from build123d import *

# Parameters (mm, degrees)
SWEEP1_PROFILE_R     = 13.49375
CUT_SWEEP1_PROFILE_R = 9.525


with BuildPart() as part:
    # Sweep1: sweep along a curve in space
    with BuildLine() as sweep1_path:
        Line((-39.450636639, 0, 30.750046958), (-39.450636639, 0, 11.700046958))
        Line((-39.450636639, 0, 0), (-39.450636639, 0, 11.700046958))
        Line((-39.450636639, 0, -7.349953042), (-39.450636639, 0, 0))
        ThreePointArc((-39.450636639, 0, -7.349953042), (-28.291405002, 0, -34.290721405), (-1.350636639, 0, -45.449953042))
        Line((-1.350636639, 0, -45.449953042), (24.049363361, 0, -45.449953042))
    # Sweep1 profile (on start of the path) → Sweep1 (sweep)
    with BuildSketch(Plane(origin=(-39.450636639, 0, 30.750046958), x_dir=(-1, 0, 0), z_dir=(0, 0, -1))):
        Circle(SWEEP1_PROFILE_R)
    sweep(path=sweep1_path.line)

    # Cut-Sweep1: sweep along a curve in space
    with BuildLine() as cut_sweep1_path:
        Line((-39.450636639, 0, 30.750046958), (-39.450636639, 0, 11.700046958))
        Line((-39.450636639, 0, 0), (-39.450636639, 0, 11.700046958))
        Line((-39.450636639, 0, -7.349953042), (-39.450636639, 0, 0))
        ThreePointArc((-39.450636639, 0, -7.349953042), (-28.291405002, 0, -34.290721405), (-1.350636639, 0, -45.449953042))
        Line((-1.350636639, 0, -45.449953042), (24.049363361, 0, -45.449953042))
    # Cut-Sweep1 profile (on start of the path) → Cut-Sweep1 (sweep, cut)
    with BuildSketch(Plane(origin=(-39.450636639, 0, 30.750046958), x_dir=(-1, 0, 0), z_dir=(0, 0, -1))):
        Circle(CUT_SWEEP1_PROFILE_R)
    sweep(path=cut_sweep1_path.line, mode=Mode.SUBTRACT)


solid = part.part
Verification items for the finished model (mm, model axes). A direction names the side the tool comes from. Coordinates: 2 decimals unless noted, no trailing zeros.
Item 1: Depth check by flat-ended pin: pin 1 (1.5 mm diameter, centred on x = -26.5, z = -40, fed in from +Y); pin 2 (6 mm diameter, centred on x = -34.5, y = -9, fed in from -Z); pin 3 (2 mm diameter, centred on x = 14.5, y = 5.5, fed in from +Z). Enter the tip coordinate at first touch or a pass-through.
Filled in:
pin 1: stops at y = 13.29
pin 2: stops at z = -46.19
pin 3: stops at z = -32.73
Item 2: Access from +Z, -Z, +X, -X, +Y, -Y to the whole of each face (thin tool, end or side, straight path). Record for faces 5 (the face through (24.049, 3, -55)), 6 (the face through (-52.321, 4.053, 11.433)).
Filled in:
face 5: +Z, -Z, +X, +Y, -Y
face 6: +Z
Item 3: Material ranges on L1, parallel to Z at x = 7, y = 0; L2, parallel to X at y = -0.5, z = 13.5; L3, parallel to X at y = 1.75, z = 3.5, recorded low to high.
Filled in:
L1: z = -58.94 to -54.97, -35.92 to -31.96
L2: x = -52.94 to -48.96, -29.94 to -25.97
L3: x = -52.83 to -48.81, -30.09 to -26.07
Item 4: Release check for a two-part mould opening along Z. For faces 1 (the face through (-30, -3, 30.75)), 2 (the face through (11.53, 0.59, -31.97)), 3 (the face through (11.53, -3.65, -54.25)), 4 (the face through (-37.4, -9.3, 11.4)) record: +Z half, -Z half, draft (parallel to the pull), parting line (faces both ways), or undercut.
Filled in:
face 1: +Z half
face 2: parting line
face 3: undercut
face 4: draft
